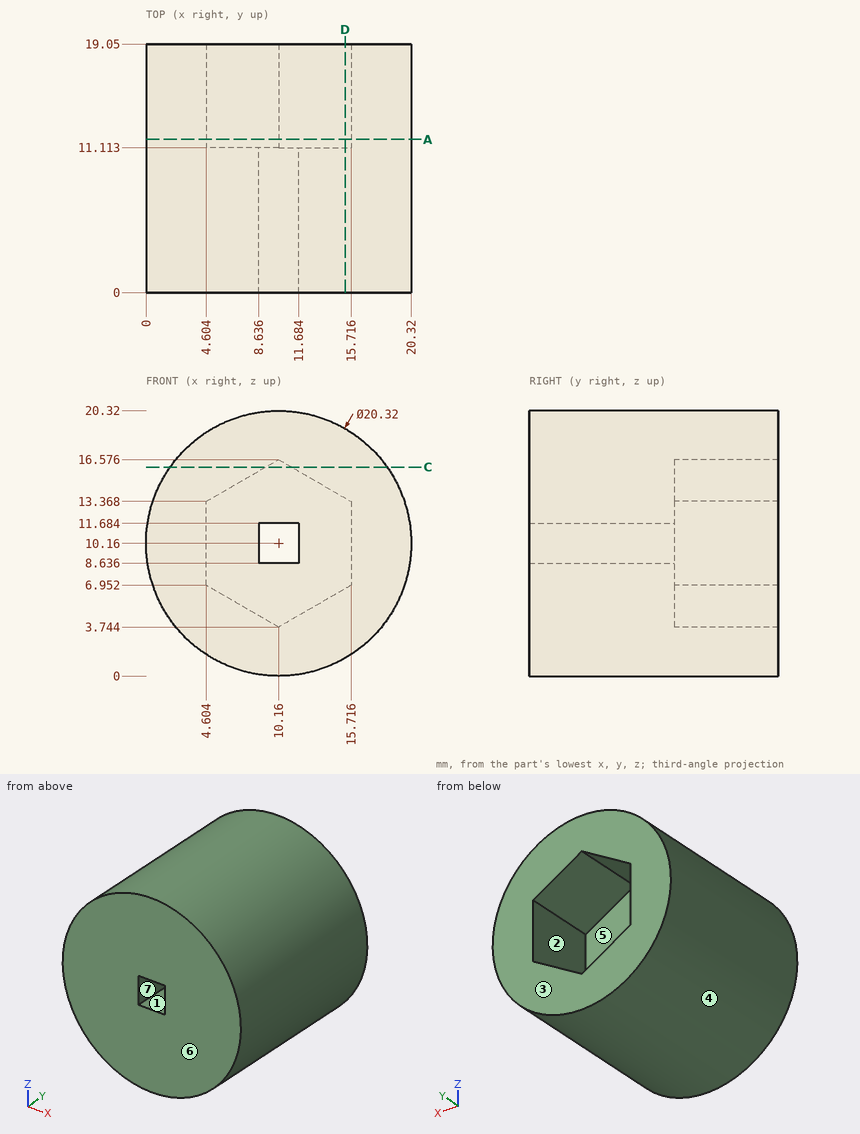
Source: three-view drawing plus pictorial views. Frame: mm from the lowest corner of the part. A direction names the side the tool comes from. Coordinates: 2 decimals unless noted, no trailing zeros. Write each loop counter-clockwise with the first axis right and the second up, starting at its lowest first coordinate (ties: lowest second). Pieces come first, ordered by that corner, then holes. Notation, with made-up numbers: (44.5, 35) - (52.5, 35) arc R19 ccw to (52.5, 60) - close; hole circle Ø5 at (4, 85). An arc over 180 degrees is marked (long way). Answer as a JSON object with one key per item and string values.
Q1. Section query C-C, the plane z = 16. Output: boundary loops of the cut face in (x, y).
Ans:
{"outline": "(1.85, 0) - (18.47, 0) - (18.47, 19.05) - (11.16, 19.05) - (11.16, 11.11) - (9.16, 11.11) - (9.16, 19.05) - (1.85, 19.05) - close"}
Q2. Draft query along Z for the marked faces 4, 5, 6 and 7. Return one class per face: released by +Z, released by -Z, zero draft, split by the parting line, or undercut.
Ans:
{"face 4": "split by the parting line", "face 5": "undercut", "face 6": "zero draft", "face 7": "undercut"}
Q3. Section query D-D, the plane x = 15.25. Output: boundary loops of the cut face in (y, z), plus the area to 3 significant figures.
Ans:
{"outline": "(0, 1.37) - (19.05, 1.37) - (19.05, 6.68) - (11.11, 6.68) - (11.11, 13.64) - (19.05, 13.64) - (19.05, 18.95) - (0, 18.95) - close", "area": "280 mm2"}
Q4. Set-up query: the marked faces 1, 2 and 3. Return all of +Z, -Z, +X, -X, +Y, -Y with unobstructed straight access to the full face (end or side cutting, diameter ignored); none if empty.
Ans:
{"face 1": "+Y, -Y", "face 2": "+Y", "face 3": "+Z, -Z, +X, -X, +Y"}
Q5. First-contact query: pin 1 Ø4 at (y, z) = (2.5, 6.5) entering from +X; pin 2 Ø2 at (y, z) = (16.5, 4.5) entering from -X; pin 3 Ø1.9 at (y, z) = (15.5, 11.5) entering from +X. Flat tips, straight axial feed; report the tip coordinate or a pass-through.
Ans:
{"pin 1": "stops at x = 20.18", "pin 2": "stops at x = 1.13", "pin 3": "stops at x = 20.31"}
Q6. Material intervals for line 1 (Z direction, x = 10, y = 6.25) (1 decimal); line 2 (X direction, y = 14, z = 5.75) (1 decimal); line 3 (Z direction, x = 13, y = 11.75) (1 decimal), sorted ascending. Write a range as [from, to].
Ans:
{"line 1": "z = [0, 8.6], [11.7, 20.3]", "line 2": "x = [1, 6.7], [13.6, 19.3]", "line 3": "z = [0.4, 5.4], [14.9, 19.9]"}
Q7. Section query A-A, the plane y = 11.75. Output: boundary loops of the cut face in (x, z) (1 decimal).
Ans:
{"outline": "circle Ø20.3 at (10.2, 10.2); hole (4.6, 7) - (10.2, 3.7) - (15.7, 7) - (15.7, 13.4) - (10.2, 16.6) - (4.6, 13.4) - close"}
